Can you work these out from the model? Positions are in its coordinate system, mm. A direction names the side the tool comes from. Round coordinates to 2 decimals unless told otherwise and drop trailing zeros. Order: outer loops, then holes, each group sorted by start corner. A loop starts at its lowest first (then second) coordinate and runs counter-clockwise, first axis right, second up. Notation, with made-up numbers: (62, -14) - (88, -14) arc R27 ccw to (88, 7) - close; hole circle Ø2 at (86, -25). An arc over 180 degrees is marked (long way). Write item = value, one per line.
from build123d import *

# Parameters (mm, degrees)
SKETCH_1_W          = 22
SKETCH_1_H          = 6
SKETCH_1_W_2        = 6
SKETCH_1_H_2        = 22
SKETCH_1_R          = 1.5
EXTRUDE_1_DEPTH     = 2
SKETCH_2_R          = 1.15
CUT_EXTRUDE_1_DEPTH = 12
CHAMFER_1_SIZE      = 8


with BuildPart() as part:
    # 草图1 → 凸台-拉伸1 (new body)
    # profile 1 of 5: a face of its own
    with BuildSketch(Plane(origin=(0, 0, 0), x_dir=(1, 0, 0), z_dir=(0, 1, 0))):
        with Locations((-14, 0)):
            Rectangle(SKETCH_1_W, SKETCH_1_H)
    # profile 2 of 5: a face of its own
    with BuildSketch(Plane(origin=(0, 0, 0), x_dir=(1, 0, 0), z_dir=(0, 1, 0))):
        with Locations((14, 0)):
            Rectangle(SKETCH_1_W, SKETCH_1_H)
    # profile 3 of 5: a face of its own
    with BuildSketch(Plane(origin=(0, 0, 0), x_dir=(1, 0, 0), z_dir=(0, 1, 0))):
        with Locations((0, 14)):
            Rectangle(SKETCH_1_W_2, SKETCH_1_H_2)
    # profile 4 of 5: a face of its own
    with BuildSketch(Plane(origin=(0, 0, 0), x_dir=(1, 0, 0), z_dir=(0, 1, 0))):
        with Locations((0, -14)):
            Rectangle(SKETCH_1_W_2, SKETCH_1_H_2)
    # profile 5 of 5: a face of its own
    with BuildSketch(Plane(origin=(0, 0, 0), x_dir=(1, 0, 0), z_dir=(0, 1, 0))):
        Rectangle(SKETCH_1_W_2, SKETCH_1_H)
        with Locations(Location((0, 0, 0), (0, 0, 270))):
            Circle(SKETCH_1_R, mode=Mode.SUBTRACT)
    extrude(amount=EXTRUDE_1_DEPTH)

    # 草图2 → 切除-拉伸1 (cut)
    with BuildSketch(Plane(origin=(0, 2, 0), x_dir=(1, 0, 0), z_dir=(0, 1, 0))):
        with Locations(Location((0, 10.5, 0), (0, 0, 270))):
            Circle(SKETCH_2_R)
        with Locations(Location((0, 16.5, 0), (0, 0, 270))):
            Circle(SKETCH_2_R)
        with Locations(Location((16.5, 0, 0), (0, 0, 270))):
            Circle(SKETCH_2_R)
        with Locations(Location((10.5, 0, 0), (0, 0, 270))):
            Circle(SKETCH_2_R)
        with Locations(Location((0, -16.5, 0), (0, 0, 270))):
            Circle(SKETCH_2_R)
        with Locations(Location((0, -10.5, 0), (0, 0, 270))):
            Circle(SKETCH_2_R)
        with Locations(Location((-16.5, 0, 0), (0, 0, 270))):
            Circle(SKETCH_2_R)
        with Locations(Location((-10.5, 0, 0), (0, 0, 270))):
            Circle(SKETCH_2_R)
    extrude(amount=-CUT_EXTRUDE_1_DEPTH, mode=Mode.SUBTRACT)

    # 倒角1
    chamfer_1_edges = [part.edges().sort_by_distance(p)[0] for p in [
        (-3, 1, -3),
        (3, 1, -3),
        (3, 1, 3),
        (-3, 1, 3),
    ]]
    chamfer(chamfer_1_edges, length=CHAMFER_1_SIZE)


solid = part.part
(1) On a 3-axis mill with a long thin cutter (end or side, diameter ignored), from which of +Z, -Z, +X, -X, +Y, -Y can I reach the whole of each face in a straight line? I mean faces 5 (the face through (0.05, 1.01, -17.65)), 6 (the face through (-18, 1, -3)), 7 (the face through (18, 1, 3)), 8 (the face through (-3, 1, 18)). Say none if no direction works.
Computed:
face_5 = +Y, -Y
face_6 = -Z, -X, +Y, -Y
face_7 = +Z, +X, +Y, -Y
face_8 = +Z, -X, +Y, -Y
(2) If we section it at A-A (x = 16.5): Write out the boundary of the cut face in (y, z).
Computed:
outline = (0, -3) - (2, -3) - (2, -1.15) - (0, -1.15) - close; (0, 1.15) - (2, 1.15) - (2, 3) - (0, 3) - close
(3) Thinking about a two-plate mould opening in Z: for faces 1 (the face through (0, 2, -2)), 2 (the face through (-17.52, 1.01, 0.53)), 3 (the face through (0.45, 0.99, 1.43)), 4 (the face through (-7, 1, -7)), which applies, +Z half, -Z half, draft (parallel to the pull), parting line (faces both ways), or undercut?
Computed:
face_1 = draft
face_2 = undercut
face_3 = undercut
face_4 = -Z half
(4) If we section it at D-D (z = 0): Write out the boundary of the cut face in (x, y), plus the area to 3 significant figures.
Computed:
outline = (-25, 0) - (-17.65, 0) - (-17.65, 2) - (-25, 2) - close; (-15.35, 0) - (-11.65, 0) - (-11.65, 2) - (-15.35, 2) - close; (-9.35, 0) - (-1.5, 0) - (-1.5, 2) - (-9.35, 2) - close; (1.5, 0) - (9.35, 0) - (9.35, 2) - (1.5, 2) - close; (11.65, 0) - (15.35, 0) - (15.35, 2) - (11.65, 2) - close; (17.65, 0) - (25, 0) - (25, 2) - (17.65, 2) - close
area = 75.6 mm^2
(5) If I drill on line 1 (X direction, y = 0.5, z = 0); line 2 (X direction, y = 1.2, z = 16.5); line 3 (X direction, y = 0.8, z = 10), over which ranges is the centre line in solid material (lowest first)? Write a range as from..to.
Computed:
line_1 = -25..-17.65, -15.35..-11.65, -9.35..-1.5, 1.5..9.35, 11.65..15.35, 17.65..25
line_2 = -3..-1.15, 1.15..3
line_3 = -4..-1.04, 1.04..4
(6) If we section it at B-B (z = -16.5): Write out the boundary of the cut face in (x, y).
Computed:
outline = (-3, 0) - (-1.15, 0) - (-1.15, 2) - (-3, 2) - close; (1.15, 0) - (3, 0) - (3, 2) - (1.15, 2) - close
(7) Will these pins go through, and if not, where does the flat tip stop? P1, Ø1, axis at x = 14.5, y = 1, coming from the +Z side; P2, Ø1, axis at y = 1.5, z = -17, coming from the -X side; P3, Ø0.6, axis at y = 0.5, z = -19, coming from the +X side; P4, Ø1.8, axis at x = 10.5, z = 0, coming from the -Y side.
Computed:
P1 = 3
P2 = -3
P3 = 3
P4 = through
(8) If we section it at C-C (y = 1.1): State how many separate pieces and enclosed holes the cut face has, plus the area to 3 significant figures.
Computed:
separate_pieces = 1
enclosed_holes = 9
area = 652 mm^2
